```python
from build123d import *

# Parameters (mm, degrees)
SKETCH1_W           = 160
SKETCH1_H           = 120
BOSS_EXTRUDE1_DEPTH = 3
SKETCH2_R           = 5
CUT_EXTRUDE1_DEPTH  = 2
SKETCH3_W           = 42
SKETCH3_H           = 42
CUT_EXTRUDE2_DEPTH  = 2
CUT_EXTRUDE3_DEPTH  = 1
BOSS_EXTRUDE2_DEPTH = 20
BOSS_EXTRUDE3_DEPTH = 1
SKETCH7_W           = 60
SKETCH7_H           = 60
CUT_EXTRUDE4_DEPTH  = 20
CUT_EXTRUDE5_REACH  = 120.258
SKETCH8_W           = 54
SKETCH8_H           = 15
BOSS_EXTRUDE4_DEPTH = 120
BOSS_EXTRUDE5_DEPTH = 3
SKETCH11_W          = 3
SKETCH11_H          = 35
BOSS_EXTRUDE6_DEPTH = 10


with BuildPart() as part:
    # Sketch1 → Boss-Extrude1 (new body)
    with BuildSketch(Plane(origin=(0, 0, 0), x_dir=(1, 0, 0), z_dir=(0, 1, 0))):
        Rectangle(SKETCH1_W, SKETCH1_H)
    extrude(amount=BOSS_EXTRUDE1_DEPTH)

    # Sketch2 → Cut-Extrude1 (cut)
    with BuildSketch(Plane.XZ):
        with Locations(Location((-70, 50, 0), (0, 0, 270))):
            Circle(SKETCH2_R)
        with Locations(Location((0, 50, 0), (0, 0, 270))):
            Circle(SKETCH2_R)
        with Locations(Location((70, 50, 0), (0, 0, 270))):
            Circle(SKETCH2_R)
        with Locations(Location((-70, 0, 0), (0, 0, 270))):
            Circle(SKETCH2_R)
        with Locations(Location((70, 0, 0), (0, 0, 270))):
            Circle(SKETCH2_R)
        with Locations(Location((-70, -50, 0), (0, 0, 270))):
            Circle(SKETCH2_R)
        with Locations(Location((0, -50, 0), (0, 0, 270))):
            Circle(SKETCH2_R)
        with Locations(Location((70, -50, 0), (0, 0, 270))):
            Circle(SKETCH2_R)
    extrude(amount=-CUT_EXTRUDE1_DEPTH, mode=Mode.SUBTRACT)

    # Sketch3 → Cut-Extrude2 (cut)
    with BuildSketch(Plane.XZ):
        with Locations((-32, 12)):
            Rectangle(SKETCH3_W, SKETCH3_H)
    extrude(amount=-CUT_EXTRUDE2_DEPTH, mode=Mode.SUBTRACT)

    # Sketch4 → Cut-Extrude3 (cut)
    with BuildSketch(Plane.XZ.offset(-2)):
        Polygon((-46, 33), (-18, 33), (-18, 26), (-11, 26), (-11, -2), (-18, -2), (-18, -9), (-46, -9), (-46, -2), (-53, -2), (-53, 26), (-46, 26), align=None)
    extrude(amount=-CUT_EXTRUDE3_DEPTH, mode=Mode.SUBTRACT)

    # Sketch5 → Boss-Extrude2 (add)
    with BuildSketch(Plane(origin=(0, 3, 0), x_dir=(1, 0, 0), z_dir=(0, 1, 0))):
        Polygon((0, 40), (-32, 40), (-32, -24), (32, -24), (32, 40), align=None)
    extrude(amount=BOSS_EXTRUDE2_DEPTH)

    # Sketch6 → Boss-Extrude3 (add)
    with BuildSketch(Plane.XZ.offset(-3)):
        Polygon((-32, 24), (-11, 24), (-11, -2), (-18, -2), (-18, -9), (-32, -9), align=None)
    extrude(amount=BOSS_EXTRUDE3_DEPTH)

    # Sketch7 → Cut-Extrude4 (cut)
    with BuildSketch(Plane(origin=(0, 23, 0), x_dir=(1, 0, 0), z_dir=(0, 1, 0))):
        with Locations((0, 8)):
            Rectangle(SKETCH7_W, SKETCH7_H)
    extrude(amount=-CUT_EXTRUDE4_DEPTH, mode=Mode.SUBTRACT)

    # Sketch8 → Cut-Extrude5 (cut, up to next)
    with BuildSketch(Plane.XY.offset(24), mode=Mode.PRIVATE) as cut_extrude5_sk1:
        with Locations((0, 10.5)):
            Rectangle(SKETCH8_W, SKETCH8_H)
    cut_extrude5_tool1 = extrude(cut_extrude5_sk1.sketch, amount=-CUT_EXTRUDE5_REACH, mode=Mode.PRIVATE) & part.part
    add(cut_extrude5_tool1.solids().sort_by_distance((0, 10.5, 24))[0], mode=Mode.SUBTRACT)

    # Sketch9 → Boss-Extrude4 (add)
    with BuildSketch(Plane(origin=(0, 3, 0), x_dir=(1, 0, 0), z_dir=(0, 1, 0))):
        Polygon((0, -24), (5, -24), (5, -34), (-5, -34), (-5, -24), align=None)
    extrude(amount=BOSS_EXTRUDE4_DEPTH)

    # Sketch10 → Boss-Extrude5 (add)
    with BuildSketch(Plane(origin=(0, 123, 0), x_dir=(1, 0, 0), z_dir=(0, 1, 0))):
        Polygon((0, -34), (25.5, -34), (25.5, 1), (-27.5, 1), (-27.5, -34), align=None)
    extrude(amount=BOSS_EXTRUDE5_DEPTH)

    # Sketch11 → Boss-Extrude6 (add)
    with BuildSketch(Plane(origin=(0, 126, 0), x_dir=(1, 0, 0), z_dir=(0, 1, 0))):
        with Locations((24, -16.5)):
            Rectangle(SKETCH11_W, SKETCH11_H)
        with Locations((-26, -16.5)):
            Rectangle(SKETCH11_W, SKETCH11_H)
    extrude(amount=BOSS_EXTRUDE6_DEPTH)


solid = part.part
```
Model file for the job. Use its own axes, mm. A direction names the side the tool comes from. Give positions to 0.01 mm unless a question says otherwise; leave off trailing zeros. Write each loop counter-clockwise with the first axis right and the second up, starting at its lowest first coordinate (ties: lowest second). Pieces come first, ordered by that corner, then holes. Notation, with made-up numbers: (-39, 13) -> (7, 13) arc R14 ccw to (7, 17) -> close; hole circle Ø11 at (73.5, -25.75). An arc over 180 degrees is marked (long way). Use CSV: the item, a comma, the result in double quotes. Start each with the question number.
1) Cut at B-B on z = -32. List the corners of the cut face in (x, y).
2) Pin check, flat tips, straight feed: P1, Ø3, axis at x = 7, y = 74.5, coming from the -Z side; P2, Ø2, axis at x = -50.5, z = -6, coming from the -Y side; P3, Ø5, axis at x = -45.5, z = 24, coming from the +Y side; P4, Ø11, axis at x = 2.5, y = 49.5, coming from the -Z side. Stop position of each tip, or through.
3) Cut at C-C on x = -70. List the corners of the cut face in (y, z), plus the area to 3 significant figures.
4) Tool access for faces 1 (the flat face through (-24.5, 131, 17)), 2 (the flat face through (-3, 125, -1)), 3 (the flat face through (0, 10, 24)): list every direction of +Z, -Z, +X, -X, +Y, -Y with a clear straight run to the whole face (end or side of a thin tool).
5) Cut at A-A on x = 8.5. List the corners of the cut face in (y, z).
6) Cut at D-D on z = -50. List the corners of the cut face in (x, y).
7) Drill centre lines: L1, parallel to Y at x = 41, z = -19; L2, parallel to X at y = 15, z = -21.5; L3, parallel to X at y = 65, z = 30.5. Where is each one in solid material? Low to high.
8) Two-plate mould, pull along Z, no slides. Class faces 4 (the cylindrical face through (0, 1, 55)), 5 (the flat face through (24, 20, 24)), 6 (the flat face through (-1, 123, 16)): released by +Z, released by -Z, zero draft, split by the parting line, or undercut.
Final values:
1,outline,"(-80, 0) -> (80, 0) -> (80, 3) -> (32, 3) -> (32, 23) -> (30, 23) -> (30, 3) -> (-30, 3) -> (-30, 23) -> (-32, 23) -> (-32, 3) -> (-80, 3) -> close"
2,P1,"passes through"
2,P2,"stops at y = 2"
2,P3,"stops at y = 3"
2,P4,"stops at z = 24"
3,outline,"(0, -60) -> (3, -60) -> (3, 60) -> (0, 60) -> (0, 55) -> (2, 55) -> (2, 45) -> (0, 45) -> (0, 5) -> (2, 5) -> (2, -5) -> (0, -5) -> (0, -45) -> (2, -45) -> (2, -55) -> (0, -55) -> close"
3,area,"300 mm2"
4,face 1,"+Z, -Z, +Y"
4,face 2,"-Z, +X, -X, +Y"
4,face 3,"none"
5,outline,"(0, -60) -> (3, -60) -> (3, -40) -> (23, -40) -> (23, -38) -> (3, -38) -> (3, 60) -> (0, 60) -> close; (18, 22) -> (23, 22) -> (23, 24) -> (18, 24) -> close; (123, -1) -> (126, -1) -> (126, 34) -> (123, 34) -> close"
6,outline,"(-80, 0) -> (-75, 0) -> (-75, 2) -> (-65, 2) -> (-65, 0) -> (-5, 0) -> (-5, 2) -> (5, 2) -> (5, 0) -> (65, 0) -> (65, 2) -> (75, 2) -> (75, 0) -> (80, 0) -> (80, 3) -> (-80, 3) -> close"
7,L1,"y = 0 to 3"
7,L2,"x = -32 to -30, 30 to 32"
7,L3,"x = -5 to 5"
8,face 4,"undercut"
8,face 5,"released by +Z"
8,face 6,"zero draft"
